```python
from build123d import *

# Parameters (mm, degrees)
SKETCH1_R           = 6
BOSS_EXTRUDE1_DEPTH = 20
SKETCH3_W           = 4.335084662
SKETCH3_H           = 14.058639044
CUT_EXTRUDE1_DEPTH  = 38
SKETCH4_R           = 3
CUT_EXTRUDE2_DEPTH  = 8
SKETCH5_W           = 6.88313448
SKETCH5_H           = 14.671944549
CUT_EXTRUDE3_DEPTH  = 40
BOSS_EXTRUDE3_DEPTH = 2.5
SKETCH8_W           = 20.918612023
SKETCH8_H           = 4.062773159
CUT_EXTRUDE4_DEPTH  = 12.5
SKETCH9_W           = 20
SKETCH9_H           = 12
BOSS_EXTRUDE4_DEPTH = 2.5
FILLET1_R           = 5
SKETCH10_R          = 3
CUT_EXTRUDE5_DEPTH  = 6.5
FILLET2_R           = 2.5


with BuildPart() as part:
    # Sketch1 → Boss-Extrude1 (new body)
    with BuildSketch(Plane(origin=(0, 0, 0), x_dir=(0, 0, -1), z_dir=(1, 0, 0))):
        Circle(SKETCH1_R)
    extrude(amount=BOSS_EXTRUDE1_DEPTH)

    # Sketch3 → Cut-Extrude1 (cut)
    with BuildSketch(Plane.ZY):
        with Locations((4.667542331, 0.290740447)):
            Rectangle(SKETCH3_W, SKETCH3_H)
    extrude(amount=-CUT_EXTRUDE1_DEPTH, mode=Mode.SUBTRACT)

    # Sketch4 → Cut-Extrude2 (cut)
    with BuildSketch(Plane.XY.offset(2.5)):
        with Locations((5, 0)):
            Circle(SKETCH4_R)
    extrude(amount=-CUT_EXTRUDE2_DEPTH, mode=Mode.SUBTRACT)

    # Sketch5 → Cut-Extrude3 (cut)
    with BuildSketch(Plane(origin=(0, 0, 0), x_dir=(0, 0, -1), z_dir=(1, 0, 0))):
        with Locations((5.94156724, -0.380383747)):
            Rectangle(SKETCH5_W, SKETCH5_H)
    extrude(amount=CUT_EXTRUDE3_DEPTH, mode=Mode.SUBTRACT)

    # Sketch7 → Boss-Extrude3 (add, symmetric)
    with BuildSketch(Plane.XY):
        Polygon((20, 0), (20, -6), (31.63118386, -8.340680909), (38.187356623, -4.535759216), (38.187356623, 0), (31.004497384, -3.314892174), (23.978377494, 0), align=None)
    extrude(amount=BOSS_EXTRUDE3_DEPTH, both=True)

    # Sketch8 → Cut-Extrude4 (cut, symmetric)
    with BuildSketch(Plane(origin=(0, 0, 0), x_dir=(1, 0, 0), z_dir=(0, 1, 0))):
        with Locations((9.540693988, 2.03138658)):
            Rectangle(SKETCH8_W, SKETCH8_H)
    extrude(amount=CUT_EXTRUDE4_DEPTH, both=True, mode=Mode.SUBTRACT)

    # Sketch9 → Boss-Extrude4 (add)
    with BuildSketch(Plane.XY.offset(2.5)):
        with Locations((10, 0)):
            Rectangle(SKETCH9_W, SKETCH9_H)
    extrude(amount=-BOSS_EXTRUDE4_DEPTH)

    # Fillet1
    fillet1_edges = [part.edges().sort_by_distance(p)[0] for p in [
        (0, 6, 1.25),
        (0, -6, 1.25),
        (20, 6, 1.25),
    ]]
    fillet(fillet1_edges, radius=FILLET1_R)

    # Sketch10 → Cut-Extrude5 (cut)
    with BuildSketch(Plane.XY.offset(2.5)):
        with Locations((6, 0)):
            Circle(SKETCH10_R)
    extrude(amount=-CUT_EXTRUDE5_DEPTH, mode=Mode.SUBTRACT)

    # Fillet2
    fillet2_edges = [part.edges().sort_by_distance(p)[0] for p in [
        (20, -6, -1.25),
        (20, 0, -1.25),
    ]]
    fillet(fillet2_edges, radius=FILLET2_R)


solid = part.part
```
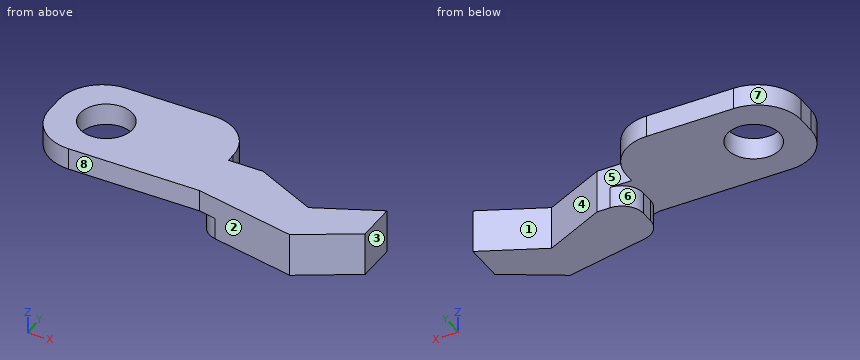
Build history of the part. All positions in model axes, mm. Face numbers are marked on the shaded views. A direction names the side the tool comes from. Round coordinates to 2 decimals unless told otherwise and drop trailing zeros. Loops run counter-clockwise (first coordinate to the right, second up) from the corner with the lowest first, then second, coordinate; pieces in that order, holes last.
Item 1: Which spindle directions (+Z, -Z, +X, -X, +Y, -Y) get a long thin tool onto all of the face, cutting with end or side? Do the marked faces 4, 5, 6, 7 and 8. Say none if no direction does.
Item 2: Saw through at B-B (y = 1.5). List the corners of the cut face in (x, z), then the cut area to 3 significant figures.
Item 3: Pin check, flat tips, straight feed: P1, Ø1.3, axis at x = 16, z = 1.5, coming from the -Y side; P2, Ø1.2, axis at x = 21, z = -1, coming from the +Y side; P3, Ø8, axis at x = 6, y = 0, coming from the -Z side. Stop position of each tip, or through.
Item 4: Drill centre lines: line 1 along Y through (x, z) = (6, 1.4); line 2 along Z through (x, y) = (14, -1); line 3 along Y through (x, z) = (22, 0.15). Where is each one in solid material? Low to high.
Item 5: Saw through at D-D (z = 1.25). List the corners of the cut face in (x, y), then the cut area to 3 significant figures.
Item 6: Two-plate mould, pull along X, no slides. Class the marked faces 1, 2 and 3: released by +X, released by -X, zero draft, split by the parting line, or undercut.
Item 7: Saw through at A-A (x = 6). List the corners of the cut face in (y, z).
Item 8: Saw through at C-C (z = -1.75). List the corners of the cut face in (x, y).
Worked answers:
1. face 4: +Z, -Z, +Y
1. face 5: +Z, -Z, +X, +Y
1. face 6: -Z, -X, +Y
1. face 7: +Z, -Z, -X, +Y
1. face 8: +Z, -Z, -X, -Y
2. outline: (0.03, 0) - (3.4, 0) - (3.4, 2.5) - (0.03, 2.5) - close; (8.6, 0) - (19.97, 0) - (19.97, 2.5) - (8.6, 2.5) - close
2. area: 36.9 mm2
3. P1: stops at y = -6
3. P2: stops at y = -0.17
3. P3: stops at z = 0
4. line 1: y = -6 to -3, 3 to 6
4. line 2: z = 0 to 2.5
4. line 3: y = -6.4 to 0
5. outline: (0, -1) arc R5 ccw to (5, -6) - (20, -6) - (31.63, -8.34) - (38.19, -4.54) - (38.19, 0) - (31, -3.31) - (23.98, 0) - (20, 0) - (20, 1) arc R5 ccw to (15, 6) - (5, 6) arc R5 ccw to (0, 1) - close; hole circle Ø6 at (6, 0)
5. area: 298 mm2
6. face 1: undercut
6. face 2: released by -X
6. face 3: released by +X
7. outline: (-6, 0) - (-3, 0) - (-3, 2.5) - (-6, 2.5) - close; (3, 0) - (6, 0) - (6, 2.5) - (3, 2.5) - close
8. outline: (20, -3.95) arc R2.5 ccw to (22.01, -6.4) - (31.63, -8.34) - (38.19, -4.54) - (38.19, 0) - (31, -3.31) - (23.98, 0) - (22.5, 0) arc R2.5 ccw to (20, -2.5) - close
